Input: part model. Units: mm. Frame: model coordinates. A direction names the side the tool comes from. Round coordinates to 2 decimals unless told otherwise and drop trailing zeros. Loops run counter-clockwise (first coordinate to the right, second up) from the corner with the lowest first, then second, coordinate; pieces in that order, holes last.
1) Draft query along X for faces 3 (the face through (31.76, -1.52, -31.88)), 4 (the face through (-31.88, -1.52, -31.76)), 5 (the face through (-2, 0, -39)). Return one class per face: pulls with the +X half, pulls with the -X half, needs draft (parallel to the pull), parting line crosses it, or undercut.
2) Ray query, line 1 along Z through (x, y) = (-36, -2.2); line 2 along X through (y, z) = (-0.7, -36); line 3 along X through (y, z) = (-0.45, -8). Return the intervals inside material, ascending.
3) First-contact query: pin 1 (1.6 mm diameter, centred on y = -1.5, z = 45.5, fed in from -X); pin 2 (0.6 mm diameter, centred on y = -1, z = -44, fed in from -X); pin 3 (4 mm diameter, centred on x = -36, z = 36, fed in from -Y); pin 4 (0.6 mm diameter, centred on y = -1.5, z = 46.5, fed in from +X). Flat tips, straight axial feed; report the tip coordinate or a pass-through.
4) Section A-A, the plane x = -6.5. Return loops of the section in (y, z), and give its area (3 significant figures).
5) Access query for faces 1 (the face through (-2, -3, -39)), 2 (the face through (-31.76, -1.52, 31.88)). Directions: +Z, -Z, +X, -X, +Y, -Y. A direction counts if a zero-diameter tool reaches every point of the face in a straight line with its end or side. Return the directions, or none.
6) Section B-B, the plane y = -0.9. State how many separate pieces and enclosed holes the cut face has, and give its area (3 significant figures).
from build123d import *

# Parameters (mm, degrees)
F0_W     = 240
F0_H     = 94
F1_DEPTH = 3
F2_W     = 5
F2_H     = 2
F2_W_2   = 230
F3_DEPTH = 25
F5_DEPTH = 25


with BuildPart() as f1:
    # F0 (on Front) → F1 (new body)
    with BuildSketch(Plane.XZ):
        Rectangle(F0_W, F0_H)
    extrude(amount=F1_DEPTH)

    # F2 (on face) → F3 (cut)
    with BuildSketch(Plane.XZ.offset(3)):
        with Locations((-117.5, 46)):
            Rectangle(F2_W, F2_H)
        Polygon((-120, -43), (-120, -47), (-115, -47), (-115, -45), (-115, -43), align=None)
        with Locations((0, -46)):
            Rectangle(F2_W_2, F2_H)
        Polygon((115, -45), (115, -47), (120, -47), (120, -43), (115, -43), align=None)
        with Locations((117.5, 46)):
            Rectangle(F2_W, F2_H)
    extrude(amount=-F3_DEPTH, mode=Mode.SUBTRACT)

    # F4 (on face) → F5 (cut)
    with BuildSketch(Plane.XZ.offset(3)):
        with BuildLine():
            Line((-36, 36), (-36, 33.85))
            ThreePointArc((-36, 33.85), (-34.47972, 34.47972), (-33.85, 36))
            Line((-33.85, 36), (-36, 36))
        make_face()
        with BuildLine():
            ThreePointArc((-33.85, 36), (-37.52028, 37.52028), (-36, 33.85))
            Line((-36, 33.85), (-36, 36))
            Line((-36, 36), (-33.85, 36))
        make_face()
        with BuildLine():
            Line((36, 36), (36, 33.85))
            ThreePointArc((36, 33.85), (37.52028, 34.47972), (38.15, 36))
            ThreePointArc((38.15, 36), (36, 38.15), (33.85, 36))
            Line((33.85, 36), (36, 36))
        make_face()
        with BuildLine():
            ThreePointArc((33.85, 36), (34.47972, 34.47972), (36, 33.85))
            Line((36, 33.85), (36, 36))
            Line((36, 36), (33.85, 36))
        make_face()
        with BuildLine():
            Line((36, -33.85), (36, -36))
            Line((36, -36), (33.85, -36))
            ThreePointArc((33.85, -36), (36, -38.15), (38.15, -36))
            ThreePointArc((38.15, -36), (37.52028, -34.47972), (36, -33.85))
        make_face()
        with BuildLine():
            Line((33.85, -36), (36, -36))
            Line((36, -36), (36, -33.85))
            ThreePointArc((36, -33.85), (34.47972, -34.47972), (33.85, -36))
        make_face()
        with BuildLine():
            ThreePointArc((-36, -33.7), (-37.626346, -37.626346), (-33.7, -36))
            Line((-33.7, -36), (-36, -36))
            Line((-36, -36), (-36, -33.7))
        make_face()
        with BuildLine():
            Line((-36, -36), (-33.7, -36))
            ThreePointArc((-33.7, -36), (-34.373654, -34.373654), (-36, -33.7))
            Line((-36, -33.7), (-36, -36))
        make_face()
        with BuildLine():
            ThreePointArc((22.793859, -38.8), (24.936261, -37.459083), (27, -36))
            ThreePointArc((27, -36), (31.819805, -31.819805), (36, -27))
            ThreePointArc((36, -27), (37.459083, -24.936261), (38.8, -22.793859))
            Line((38.8, -22.793859), (38.8, 22.793859))
            ThreePointArc((38.8, 22.793859), (37.459083, 24.936261), (36, 27))
            ThreePointArc((36, 27), (31.819805, 31.819805), (27, 36))
            ThreePointArc((27, 36), (24.936261, 37.459083), (22.793859, 38.8))
            Line((22.793859, 38.8), (-22.793859, 38.8))
            ThreePointArc((-22.793859, 38.8), (-24.936261, 37.459083), (-27, 36))
            ThreePointArc((-27, 36), (-31.819805, 31.819805), (-36, 27))
            ThreePointArc((-36, 27), (-37.459083, 24.936261), (-38.8, 22.793859))
            Line((-38.8, 22.793859), (-38.8, -22.793859))
            ThreePointArc((-38.8, -22.793859), (-37.459083, -24.936261), (-36, -27))
            ThreePointArc((-36, -27), (-31.819805, -31.819805), (-27, -36))
            ThreePointArc((-27, -36), (-24.936261, -37.459083), (-22.793859, -38.8))
            Line((-22.793859, -38.8), (22.793859, -38.8))
        make_face()
    extrude(amount=-F5_DEPTH, mode=Mode.SUBTRACT)


solid = f1.part
Final values:
1. face 3: undercut
1. face 4: undercut
1. face 5: needs draft
2. line 1: z = -45 to -38.3, -33.7 to -27, 27 to 33.85, 38.15 to 47
2. line 2: x = -120 to -38.3, -33.7 to -27, 27 to 33.85, 38.15 to 120
2. line 3: x = -120 to -38.8, 38.8 to 120
3. pin 1: stops at x = -120
3. pin 2: stops at x = -115
3. pin 3: passes through
3. pin 4: stops at x = 115
4. outline: (-3, -45) - (0, -45) - (0, -38.8) - (-3, -38.8) - close; (-3, 38.8) - (0, 38.8) - (0, 47) - (-3, 47) - close
4. area: 43.2 mm2
5. face 1: +Z, -Z, +X, -X, -Y
5. face 2: +Y, -Y
6. separate pieces: 1
6. enclosed holes: 5
6. area: 16,400 mm2
